Here's how the part is built. I have some questions about the finished solid (model axes, mm). A direction names the side the tool comes from. Round coordinates to 2 decimals unless told otherwise and drop trailing zeros. Write each loop counter-clockwise with the first axis right and the second up, starting at its lowest first coordinate (ties: lowest second). Pieces come first, ordered by that corner, then holes. Notation, with made-up numbers: (-36.75, -6) -> (-29.75, -6) arc R22 ccw to (-29.75, 22) -> close; hole circle Ø5 at (31.25, -9). An arc over 180 degrees is marked (long way). Answer as CSV lines item,"result".
from build123d import *

# Parameters (mm, degrees)
SKETCH1_W           = 419.1
SKETCH1_H           = 142.18412
BOSS_EXTRUDE1_DEPTH = 88.9
SKETCH2_R           = 119.38
CUT_EXTRUDE1_DEPTH  = 83.4009
SKETCH7_W           = 194.780719179
SKETCH7_H           = 43.63974
SKETCH7_H_2         = 50.8
CUT_EXTRUDE2_DEPTH  = 452.402640644
SKETCH4_R           = 40.386
CUT_EXTRUDE4_DEPTH  = 10
SKETCH18_R          = 25.527
CUT_EXTRUDE11_DEPTH = 23.09114
SKETCH5_R           = 27.686
CUT_EXTRUDE5_DEPTH  = 448.05209497
SKETCH8_W           = 419.1
SKETCH8_H           = 88.9
CUT_EXTRUDE6_DEPTH  = 7.85114
SKETCH9_W           = 419.1
SKETCH9_H           = 88.9
CUT_EXTRUDE7_DEPTH  = 11.94308
SKETCH10_W          = 219.202
SKETCH10_H          = 88.9
CUT_EXTRUDE8_DEPTH  = 30.48
SKETCH12_W          = 121.533574186
SKETCH12_H          = 91.9099
BOSS_EXTRUDE2_DEPTH = 25.4
SKETCH14_W          = 55.647095764
SKETCH14_H          = 91.9099
BOSS_EXTRUDE3_DEPTH = 12.7
CUT_EXTRUDE10_REACH = 447.564
SKETCH17_R          = 12.827
BOSS_EXTRUDE4_REACH = 446.193
SKETCH20_W          = 5.08
SKETCH20_H          = 38.1
SKETCH22_W          = 199.898
SKETCH22_H          = 88.9
BOSS_EXTRUDE5_DEPTH = 2.54
SKETCH24_R          = 29.21
CUT_EXTRUDE12_DEPTH = 2.54
CUT_EXTRUDE13_START = -5.08
SKETCH24_4_R        = 29.21
CUT_EXTRUDE13_DEPTH = 2.55016
SKETCH29_R          = 12.827
CUT_EXTRUDE14_DEPTH = 446.564033133
BOSS_EXTRUDE6_DEPTH = 86.10092


with BuildPart() as part:
    # Sketch1 → Boss-Extrude1 (new body)
    with BuildSketch(Plane(origin=(0, 0, 0), x_dir=(1, 0, 0), z_dir=(0, 1, 0))):
        with Locations((209.55, 71.09206)):
            Rectangle(SKETCH1_W, SKETCH1_H)
    extrude(amount=BOSS_EXTRUDE1_DEPTH)

    # Sketch2 → Cut-Extrude1 (cut)
    with BuildSketch(Plane(origin=(0, 0, -131.63296), x_dir=(-1, 0, 0), z_dir=(0, 0, -1))):
        with Locations((-116.7166499, 150.061217688)):
            Circle(SKETCH2_R)
    extrude(amount=-CUT_EXTRUDE1_DEPTH, mode=Mode.SUBTRACT)

    # Sketch7 → Cut-Extrude2 (cut, through all)
    with BuildSketch(Plane(origin=(0, 88.9, 0), x_dir=(1, 0, 0), z_dir=(0, 1, 0))):
        with Locations((321.709640411, 97.27311)):
            Rectangle(SKETCH7_W, SKETCH7_H)
        with Locations((321.709640411, 42.43324)):
            Rectangle(SKETCH7_W, SKETCH7_H_2)
    extrude(amount=-CUT_EXTRUDE2_DEPTH, mode=Mode.SUBTRACT)

    # Sketch4 → Cut-Extrude4 (cut)
    with BuildSketch(Plane(origin=(0, 0, -67.83324), x_dir=(-1, 0, 0), z_dir=(0, 0, -1))):
        with Locations((-278.649352085, 104.852009966)):
            Circle(SKETCH4_R)
    extrude(amount=CUT_EXTRUDE4_DEPTH, mode=Mode.SUBTRACT)

    # Sketch18 → Cut-Extrude11 (cut)
    with BuildSketch(Plane(origin=(0, 0, -142.18412), x_dir=(-1, 0, 0), z_dir=(0, 0, -1))):
        with Locations((-278.649352085, 104.852009966)):
            Circle(SKETCH18_R)
    extrude(amount=-CUT_EXTRUDE11_DEPTH, mode=Mode.SUBTRACT)

    # Sketch5 → Cut-Extrude5 (cut, through all)
    with BuildSketch(Plane(origin=(0, 0, -14.48308), x_dir=(-1, 0, 0), z_dir=(0, 0, -1))):
        with Locations((-278.649352085, 104.852009966)):
            Circle(SKETCH5_R)
    extrude(amount=-CUT_EXTRUDE5_DEPTH, mode=Mode.SUBTRACT)

    # Sketch8 → Cut-Extrude6 (cut)
    with BuildSketch(Plane(origin=(0, 0, -142.18412), x_dir=(-1, 0, 0), z_dir=(0, 0, -1))):
        with Locations((-209.55, 44.45)):
            Rectangle(SKETCH8_W, SKETCH8_H)
    extrude(amount=-CUT_EXTRUDE6_DEPTH, mode=Mode.SUBTRACT)

    # Sketch9 → Cut-Extrude7 (cut)
    with BuildSketch(Plane.XY):
        with Locations((209.55, 44.45)):
            Rectangle(SKETCH9_W, SKETCH9_H)
    extrude(amount=-CUT_EXTRUDE7_DEPTH, mode=Mode.SUBTRACT)

    # Sketch10 → Cut-Extrude8 (cut)
    with BuildSketch(Plane.XY.offset(-11.94308)):
        with Locations((109.601, 44.45)):
            Rectangle(SKETCH10_W, SKETCH10_H)
    extrude(amount=-CUT_EXTRUDE8_DEPTH, mode=Mode.SUBTRACT)

    # Sketch12 → Boss-Extrude2 (add)
    with BuildSketch(Plane.XZ):
        with Locations((-60.766787093, -88.37803)):
            Rectangle(SKETCH12_W, SKETCH12_H)
    extrude(amount=-BOSS_EXTRUDE2_DEPTH)

    # Sketch14 → Boss-Extrude3 (add)
    with BuildSketch(Plane.XZ):
        with Locations((-93.710026304, -88.37803)):
            Rectangle(SKETCH14_W, SKETCH14_H)
    extrude(amount=BOSS_EXTRUDE3_DEPTH)

    # Cut-Extrude10: up to this face of the body (flat: up to its plane)
    cut_extrude10_end = Plane(part.part.faces().sort_by_distance((320.017892525, 43.601141034, -11.94308))[0])
    # Sketch17 → Cut-Extrude10 (cut, up to the picked face)
    with BuildSketch(Plane(origin=(0, 0, -134.33298), x_dir=(-1, 0, 0), z_dir=(0, 0, -1)), mode=Mode.PRIVATE) as cut_extrude10_sk1:
        with Locations((-384.735935495, 0.531880938)):
            Circle(SKETCH17_R)
    cut_extrude10_tool1 = split(extrude(cut_extrude10_sk1.sketch, amount=-CUT_EXTRUDE10_REACH, mode=Mode.PRIVATE), bisect_by=cut_extrude10_end, keep=Keep.BOTH, mode=Mode.PRIVATE)
    # Sketch17 → Cut-Extrude10 (cut, up to the picked face)
    with BuildSketch(Plane(origin=(0, 0, -134.33298), x_dir=(-1, 0, 0), z_dir=(0, 0, -1)), mode=Mode.PRIVATE) as cut_extrude10_sk2:
        with Locations((94.798916194, -17.274045482)):
            Circle(SKETCH17_R)
    cut_extrude10_tool2 = split(extrude(cut_extrude10_sk2.sketch, amount=-CUT_EXTRUDE10_REACH, mode=Mode.PRIVATE), bisect_by=cut_extrude10_end, keep=Keep.BOTH, mode=Mode.PRIVATE)
    # Sketch17 → Cut-Extrude10 (cut, up to the picked face)
    with BuildSketch(Plane(origin=(0, 0, -134.33298), x_dir=(-1, 0, 0), z_dir=(0, 0, -1)), mode=Mode.PRIVATE) as cut_extrude10_sk3:
        with BuildLine():
            Line((-169.736021607, 19.31637742), (-169.736021607, 0))
            Line((-169.736021607, 0), (-144.082021607, 0))
            Line((-144.082021607, 0), (-144.082021607, 19.31637742))
            ThreePointArc((-144.082021607, 19.31637742), (-156.909021607, 32.14337742), (-169.736021607, 19.31637742))
        make_face()
    cut_extrude10_tool3 = split(extrude(cut_extrude10_sk3.sketch, amount=-CUT_EXTRUDE10_REACH, mode=Mode.PRIVATE), bisect_by=cut_extrude10_end, keep=Keep.BOTH, mode=Mode.PRIVATE)
    add(cut_extrude10_tool1.solids().sort_by(Axis((384.735935, 0.531881, -134.33298), (0, 0, 1)))[0], mode=Mode.SUBTRACT)
    add(cut_extrude10_tool2.solids().sort_by(Axis((-94.798916, -17.274045, -134.33298), (0, 0, 1)))[0], mode=Mode.SUBTRACT)
    add(cut_extrude10_tool3.solids().sort_by(Axis((156.909022, 14.834778, -134.33298), (0, 0, 1)))[0], mode=Mode.SUBTRACT)

    # Boss-Extrude4: up to this face of the body (flat: up to its plane)
    boss_extrude4_end = Plane(part.part.faces().sort_by_distance((183.515144796, 41.822372775, -134.33298))[0])
    # Sketch20 → Boss-Extrude4 (add, up to the picked face)
    with BuildSketch(Plane(origin=(0, 0, -17.03324), x_dir=(-1, 0, 0), z_dir=(0, 0, -1)), mode=Mode.PRIVATE) as boss_extrude4_sk1:
        with Locations((-416.56, 31.75)):
            Rectangle(SKETCH20_W, SKETCH20_H)
    boss_extrude4_tool1 = split(extrude(boss_extrude4_sk1.sketch, amount=BOSS_EXTRUDE4_REACH, mode=Mode.PRIVATE), bisect_by=boss_extrude4_end, keep=Keep.BOTH, mode=Mode.PRIVATE)
    add(boss_extrude4_tool1.solids().sort_by(Axis((416.56, 31.75, -17.03324), (0, 0, -1)))[0])

    # Sketch22 → Boss-Extrude5 (add)
    with BuildSketch(Plane.XY.offset(-11.94308)):
        with Locations((319.151, 44.45)):
            Rectangle(SKETCH22_W, SKETCH22_H)
    extrude(amount=BOSS_EXTRUDE5_DEPTH)

    # Sketch24 → Cut-Extrude12 (cut)
    with BuildSketch(Plane.XY.offset(-9.40308)):
        with Locations((278.649352085, 104.852009966)):
            Circle(SKETCH24_R)
    extrude(amount=-CUT_EXTRUDE12_DEPTH, mode=Mode.SUBTRACT)

    # Sketch24<4> → Cut-Extrude13 (cut)
    with BuildSketch(Plane.XY.offset(-9.40308).offset(CUT_EXTRUDE13_START)):
        with Locations((278.649352085, 104.852009966)):
            Circle(SKETCH24_4_R)
    extrude(amount=-CUT_EXTRUDE13_DEPTH, mode=Mode.SUBTRACT)

    # Sketch29 → Cut-Extrude14 (cut, through all)
    with BuildSketch(Plane(origin=(0, 0, -11.94308), x_dir=(-1, 0, 0), z_dir=(0, 0, -1))):
        with Locations((-384.735935495, 0.531880938)):
            Circle(SKETCH29_R)
    extrude(amount=-CUT_EXTRUDE14_DEPTH, mode=Mode.SUBTRACT)

    # Sketch30 → Boss-Extrude6 (add)
    with BuildSketch(Plane(origin=(0, 0, -134.33298), x_dir=(-1, 0, 0), z_dir=(0, 0, -1))):
        with BuildLine():
            Line((-14.194018979, 88.9), (-20.758717893, 88.9))
            ThreePointArc((-20.758717893, 88.9), (-116.7166499, 36.269217688), (-212.674581906, 88.9))
            Line((-212.674581906, 88.9), (-219.239280821, 88.9))
            ThreePointArc((-219.239280821, 88.9), (-116.7166499, 30.681217688), (-14.194018979, 88.9))
        make_face()
    extrude(amount=-BOSS_EXTRUDE6_DEPTH)


solid = part.part
Item 1: Suppose I cut it at A-A, the plane z = -83. List the corners of the cut face in (x, y) for me, then the cut area to 3 significant figures.
Results found:
outline,"(-121.53, -12.7) -> (-106.78, -12.7) arc R12.83 cw to (-82.82, -12.7) -> (-65.89, -12.7) -> (-65.89, 0) -> (144.08, 0) -> (144.08, 19.32) arc R12.83 cw to (169.74, 19.32) -> (169.74, 0) -> (224.32, 0) -> (224.32, 88.9) -> (212.67, 88.9) arc R113.79 cw to (20.76, 88.9) -> (0, 88.9) -> (0, 25.4) -> (-121.53, 25.4) -> close; (414.02, 12.7) -> (419.1, 12.7) -> (419.1, 50.8) -> (414.02, 50.8) -> close"
area,"15,900 mm²"
Item 2: I need wall thicknesses on L1, parallel to X at y = 21, z = -64; L2, parallel to Z at x = 307, y = 37.5; L3, parallel to X at y = 14.5, z = -53. Which ranges of each line are inside material? Lowest first, please.
Results found:
L1,"x = -121.53 to 144.19, 169.63 to 224.32, 414.02 to 419.1"
L2,"z = -134.33 to -119.09, -75.45 to -67.83, -17.03 to -9.4"
L3,"x = -121.53 to 144.08, 169.74 to 224.32, 414.02 to 419.1"
Item 3: Will these pins go through, and if not, where does the flat tip stop? pin 1 (4 mm diameter, centred on x = 409, z = -73.5, fed in from -Y); pin 2 (13 mm diameter, centred on y = 61, z = -90, fed in from +X); pin 3 (1.5 mm diameter, centred on x = 415.5, z = -50, fed in from -Y).
Results found:
pin 1,"stops at y = 0"
pin 2,"stops at x = 224.32"
pin 3,"stops at y = 12.7"
Item 4: Suppose I cut it at C-C, the plane z = -29.5. List the corners of the cut face in (x, y) for me, then the cut area to 3 significant figures.
Results found:
outline,"(219.2, 0) -> (224.32, 0) -> (224.32, 88.9) -> (219.2, 88.9) -> close; (414.02, 12.7) -> (419.1, 12.7) -> (419.1, 50.8) -> (414.02, 50.8) -> close"
area,"648 mm²"
Item 5: Suppose I cut it at B-B, the plane x = 378.5. List the corners of the cut face in (y, z) for me, then the cut area to 3 significant figures.
Results found:
outline,"(11.74, -134.33) -> (88.9, -134.33) -> (88.9, -119.09) -> (11.74, -119.09) -> close; (11.74, -75.45) -> (88.9, -75.45) -> (88.9, -67.83) -> (11.74, -67.83) -> close; (11.74, -17.03) -> (88.9, -17.03) -> (88.9, -9.4) -> (11.74, -9.4) -> close"
area,"2,350 mm²"
Item 6: If we mould it in two halves opening along Z, with no side actions, what happens to faces 1 (the flat face through (279, 77, -11.943)), 2 (the flat face through (279, 77, -14.483)), 3 (the cylindrical face through (-95.02, -4.45, -89.02))? For each: pulls with the +Z half, pulls with the -Z half, needs draft (parallel to the pull), parting line crosses it, or undercut.
Results found:
face 1,"pulls with the +Z half"
face 2,"undercut"
face 3,"needs draft"
Item 7: Suppose I cut it at D-D, the plane x = -76. List the corners of the cut face in (y, z) for me.
Results found:
outline,"(-12.7, -134.33) -> (25.4, -134.33) -> (25.4, -42.42) -> (-12.7, -42.42) -> close"
Item 8: For faces 4 (the flat face through (408, 0, -127)), 5 (the cylindrical face through (278.243, 75.645, -10.655)), 6 (the cylindrical face through (278.243, 75.645, -15.74)), which set-ups out of +Z, -Z, +X, -X, +Y, -Y let a thin tool reach every point of the face, with its end or its side?
Results found:
face 4,"+Z, -Z, +X, -Y"
face 5,"+Z, +Y"
face 6,"+Y"
